from build123d import *

# Parameters (mm, degrees)
F0_W     = 20
F0_H     = 6
F0_R     = 1.483649
F1_DEPTH = 16
F2_R     = 2


with BuildPart() as f1:
    # F0 (on Top) → F1 (new body)
    with BuildSketch(Plane.XY):
        with Locations((10, 3)):
            Rectangle(F0_W, F0_H)
        with Locations((10, 3)):
            Circle(F0_R, mode=Mode.SUBTRACT)
    extrude(amount=-F1_DEPTH)

    # F2
    f2_edges = [f1.edges().sort_by_distance(p)[0] for p in [
        (20, 6, -8),
        (0, 6, -8),
        (20, 0, -8),
        (0, 0, -8),
    ]]
    fillet(f2_edges, radius=F2_R)


solid = f1.part
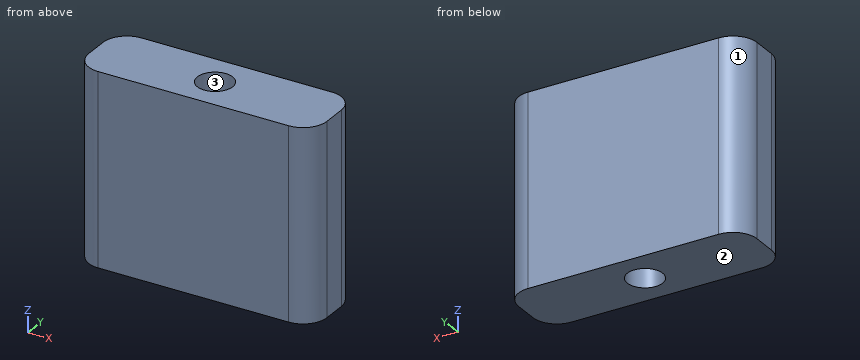
CAD build for the part. Positions are in the model's coordinates, mm. Face numbers are marked on the shaded views. Round coordinates to 2 decimals unless told otherwise and drop trailing zeros. Write each loop counter-clockwise with the first axis right and the second up, starting at its lowest first coordinate (ties: lowest second). Pieces come first, ordered by that corner, then holes. Notation, with made-up numbers: M -15.5,89 L 18.5,89 A6 ccw 18.5,95 Z; hole C -20,65.5 d2. An arc over 180 degrees is marked long. Use a Markdown table: item, result. Add a question column.
1. Slice it at D-D on y = 4.9. Give the cut face in (x, z), then the cut area to 3 significant figures.
2. Slice it at B-B on y = 3. Give the cut face in (x, z).
3. Drill centre lines: probe 1 along Y at (x, z) = (10, -4.25); probe 2 along X at (y, z) = (4.25, -2.25); probe 3 along X at (y, z) = (2.45, -7.5). Where is each one in solid material? Low to high.
4. Pull direction X, two halves, no side cores. Call the marked faces 1, 2 and 3: released by +X, released by -X, zero draft, split by the parting line, or undercut.
5. Slice it at A-A on x = 10. Give the cut face in (y, z).
6. Slice it at C-C on z = -3.75. Give the cut face in (x, y).
Reply:
| question | item | result |
|---|---|---|
| 1 | outline | M 0.21,-16 L 19.79,-16 L 19.79,0 L 0.21,0 Z |
| 1 | area | 313 mm^2 |
| 2 | outline | M 0,-16 L 8.52,-16 L 8.52,0 L 0,0 Z; M 11.48,-16 L 20,-16 L 20,0 L 11.48,0 Z |
| 3 | probe 1 | y = 0 to 1.52, 4.48 to 6 |
| 3 | probe 2 | x = 0.02 to 9.2, 10.8 to 19.98 |
| 3 | probe 3 | x = 0 to 8.62, 11.38 to 20 |
| 4 | face 1 | released by -X |
| 4 | face 2 | zero draft |
| 4 | face 3 | undercut |
| 5 | outline | M 0,-16 L 1.52,-16 L 1.52,0 L 0,0 Z; M 4.48,-16 L 6,-16 L 6,0 L 4.48,0 Z |
| 6 | outline | M 0,2 A2 ccw 2,0 L 18,0 A2 ccw 20,2 L 20,4 A2 ccw 18,6 L 2,6 A2 ccw 0,4 Z; hole C 10,3 d2.97 |
